```python
from build123d import *

# Parameters (mm, degrees)
F1_DEPTH = 3.175
F3_DEPTH = 22.225


# Not quite as in the source:
# - a feature names something its author has since deleted; it is built from what else it names


with BuildPart() as f1:
    # F0 (on Top) → F1 (new body)
    with BuildSketch(Plane.XY):
        Polygon((7.557114383, 12.7), (0, 0), (7.557114383, -12.7), (22.3354761934, -12.7), (29.8925905764, 0), (22.3354761934, 12.7), align=None)
    extrude(amount=F1_DEPTH)

    # F2 (on face) → F3 (join)
    with BuildSketch(Plane.XY.offset(3.175)):
        Polygon((7.557114383, 12.7), (0, 0), (22.3354761934, 12.7), align=None)
    extrude(amount=F3_DEPTH)


solid = f1.part
```
The listing builds one solid part. Answer for the finished solid, in the listing's coordinates (mm). A direction names the side the tool comes from. Coordinates: 2 decimals unless noted, no trailing zeros. Loops run counter-clockwise (first coordinate to the right, second up) from the corner with the lowest first, then second, coordinate; pieces in that order, holes last. Notation, with made-up numbers: M 36,52.25 L 83,52.25 A31 ccw 83,86.25 Z; hole C 88,-5 d4. An arc over 180 degrees is marked long. Answer as CSV lines item,"result". Start each with the question number.
(1) The part is cut by section D-D (z = 16.75). Give the vertices of the cut face in (x, y).
(2) Find the intervals of material crossed by L1, parallel to Z at x = 3.25, y = -3.25 (3 decimals); L2, parallel to X at y = 0.75, z = 21.5; L3, parallel to Y at x = 11.75, z = 4.25, in increasing order. Write a range as [from, to].
(3) The part is cut by section C-C (x = 26.25). Give the vertices of the cut face in (y, z) (1 decimal), and give its area (3 significant figures).
(4) The part is cut by section A-A (z = 2). Give the vertices of the cut face in (x, y), and give its area (3 significant figures).
(5) For faces 1 (the flat face through (18, -3, 3.175)), 2 (the flat face through (15, -12.7, 2)), determine the directions among +Z, -Z, +X, -X, +Y, -Y from which every point of the face is accessible in a straight line to the end or side of a thin tool.
(6) Given pin 1 (2 mm diameter, centred on x = 20, z = 9, fed in from -Y); pin 2 (2 mm diameter, centred on x = 21, y = -8.5, fed in from +Z) (3 decimals), each flat-ended and moving along its own axis, determine where each tip first touches the part or whether it passes through.
(7) The part is cut by section B-B (y = 1.25). Give the vertices of the cut face in (x, z) (3 decimals).
Determined:
1,outline,"M 0,0 L 22.34,12.7 L 7.56,12.7 Z"
2,L1,"[0, 3.175]"
2,L2,"[0.45, 1.32]"
2,L3,"[6.68, 12.7]"
3,outline,"M -6.1,0 L 6.1,0 L 6.1,3.2 L -6.1,3.2 Z"
3,area,"38.9 mm2"
4,outline,"M 0,0 L 7.56,-12.7 L 22.34,-12.7 L 29.89,0 L 22.34,12.7 L 7.56,12.7 Z"
4,area,"567 mm2"
5,face 1,"+Z, +X, -Y"
5,face 2,"+Z, -Z, +X, -X, -Y"
6,pin 1,"y = 10.8"
6,pin 2,"z = 3.175"
7,outline,"M 0.744,0 L 29.149,0 L 29.149,3.175 L 2.198,3.175 L 2.198,25.4 L 0.744,25.4 Z"
